Geometry: final body of the model. Coordinates: model frame, mm. A direction names the side the tool comes from. Give positions to 0.01 mm unless a question says otherwise; leave off trailing zeros. Loops run counter-clockwise (first coordinate to the right, second up) from the corner with the lowest first, then second, coordinate; pieces in that order, holes last. Notation, with made-up numbers: (60.5, 14.25) - (106.5, 14.25) arc R23 ccw to (106.5, 52.25) - close; hole circle Ø3 at (-39, 77). An arc over 180 degrees is marked (long way). Answer in a Markdown table with one row per item.
Autodesk Inventor part; units mm, degrees
ref_plane "YZ Plane" through (0, 0, 0) normal (1, 0, 0) x (0, 1, 0)
ref_plane "XZ Plane" through (0, 0, 0) normal (0, 1, 0) x (-1, 0, 0)
ref_plane "XY Plane" through (0, 0, 0) normal (0, 0, 1) x (1, 0, 0)
sketch "Sketch1" plane through (0, 0, 0) normal (0, 0, 1) x (1, 0, 0)
  line L0 (0, -3.15) -> (0, 3.15)
  line L1 (-1.25, 0) -> (7.5, 0)
  line L2 (4, -2.25) -> (4, 2.25)
  line L3 (4, 2.25) -> (6.25, 2.25)
  line L4 (6.25, 2.25) -> (6.25, 1.75)
  line L5 (6.25, 1.75) -> (4.5, 1.75)
  line L6 (4.5, 1.75) -> (4.5, -1.75)
  line L7 (4.5, -1.75) -> (6.25, -1.75)
  line L8 (6.25, -1.75) -> (6.25, -2.25)
  line L9 (6.25, -2.25) -> (4, -2.25)
  point P0 (0, 0)
  point P1 (4.5, 0)
  dimension "d0" = 8
  dimension "d1" = 9
  dimension "d2" = 12.5
  dimension "d3" = 0.5
  dimension "d4" = 3.5
  dimension "d5" = 0.5
revolve "Revolution1" add sketch "Sketch1" angle 360 about axis through (0, -10, 0) along (0, 1, 0)
sketch "Sketch2" plane through (0, 2.25, 0) normal (0, 1, 0) x (1, 0, 0)
  circle A0 centre (0, 0) radius 6.25
  circle A1 centre (0, 0) radius 4
  line L0 (-8.75, 0) -> (8.75, 0)
  line L1 (0, 8.75) -> (0, -8.75)
  line L2 (3.9996, -0.0535) -> (6.2164, -0.6475)
  line L3 (3.9996, 0.0535) -> (6.2164, 0.6475)
  arc A2 (3.9996, -0.0535) -> (3.9996, 0.0535) centre (0, 0) ccw
  arc A3 (6.2164, -0.6475) -> (6.2164, 0.6475) centre (0, 0) ccw
  dimension "d8" = 15
  dimension "d9" = 30
  dimension "d10" = 2.2167
  dimension "d11" = 2.2167
extrude "Extrusion1" cut sketch "Sketch2" against normal through all contours L0 A1 L3 A0 | A0 L2 A1 L0
properties part number "314-14" material "Nylon-6/6"
Q1. Cut plane A-A (z = 5). Output: boundary loops of the cut face in (x, y).
Check values:
| item | result |
|---|---|
| outline | (-3.75, -2.25) - (3.75, -2.25) - (3.75, -1.75) - (-3.75, -1.75) - close; (-3.75, 1.75) - (3.75, 1.75) - (3.75, 2.25) - (-3.75, 2.25) - close |
Q2. Cut plane D-D (x = -5.25). Output: boundary loops of the cut face in (y, z).
Check values:
| item | result |
|---|---|
| outline | (-2.25, -3.39) - (-1.75, -3.39) - (-1.75, 3.39) - (-2.25, 3.39) - close; (1.75, -3.39) - (2.25, -3.39) - (2.25, 3.39) - (1.75, 3.39) - close |
Q3. Material intervals for line 1 along Z through (x, y) = (0, 0.9); line 2 along Y through (x, z) = (-3, -3.75); line 3 along X through (y, z) = (0.9, 0.5), sorted ascending.
Check values:
| item | result |
|---|---|
| line 1 | -4.5 to -4, 4 to 4.5 |
| line 2 | -2.25 to -1.75, 1.75 to 2.25 |
| line 3 | -4.47 to -3.97, 3.97 to 4.47 |
Q4. Cut plane B-B (x = 0). Output: boundary loops of the cut face in (y, z), and give its area (3 significant figures).
Check values:
| item | result |
|---|---|
| outline | (-2.25, -6.25) - (-1.75, -6.25) - (-1.75, -4.5) - (1.75, -4.5) - (1.75, -6.25) - (2.25, -6.25) - (2.25, -4) - (-2.25, -4) - close; (-2.25, 4) - (2.25, 4) - (2.25, 6.25) - (1.75, 6.25) - (1.75, 4.5) - (-1.75, 4.5) - (-1.75, 6.25) - (-2.25, 6.25) - close |
| area | 8.00 mm² |
Q5. First-contact query: pin 1 (1.5 mm diameter, centred on x = -1, y = 0, fed in from -Z); pin 2 (1.5 mm diameter, centred on y = -0.5, z = 2.5, fed in from -X). Flat tips, straight axial feed; report the tip coordinate or a pass-through.
Check values:
| item | result |
|---|---|
| pin 1 | z = -4.49 |
| pin 2 | x = -4.15 |
Q6. Cut plane C-C (z = -3). Output: boundary loops of the cut face in (x, y).
Check values:
| item | result |
|---|---|
| outline | (-5.48, -2.25) - (-2.65, -2.25) - (-2.65, 2.25) - (-5.48, 2.25) - (-5.48, 1.75) - (-3.35, 1.75) - (-3.35, -1.75) - (-5.48, -1.75) - close; (2.65, -2.25) - (5.48, -2.25) - (5.48, -1.75) - (3.35, -1.75) - (3.35, 1.75) - (5.48, 1.75) - (5.48, 2.25) - (2.65, 2.25) - close |
Q7. Draft query along Y for faces 3 (the flat face through (-3, 2.25, -3)), 4 (the flat face through (4, 1.75, -3)), 5 (the cylindrical face through (-6.244, 1.996, 0.266)). Return one class per face: pulls with the +Y half, pulls with the -Y half, needs draft (parallel to the pull), parting line crosses it, or undercut.
Check values:
| item | result |
|---|---|
| face 3 | pulls with the +Y half |
| face 4 | undercut |
| face 5 | needs draft |
Q8. Reachability of faces 1 (the cylindrical face through (-4.496, -0.024, 0.195)), 2 (the flat face through (-3, -2.25, -3)) from +Z, -Z, +X, -X, +Y, -Y: full face, straight path, thin tool, end or side. Return the list, or none.
Check values:
| item | result |
|---|---|
| face 1 | none |
| face 2 | +Z, -Z, +X, -X, -Y |
